```python
from build123d import *

# Parameters (mm, degrees)
F1_DEPTH  = 127
F2_R      = 16.6289302691
F3_DEPTH  = 6.35
F4_W      = 2.8006685898
F4_H      = 13.494130224
F4_W_2    = 2.8006681241
F4_H_2    = 14.0033438802
F5_DEPTH  = 2.54
F6_R      = 6.3651576638
F7_DEPTH  = 3.81
F10_W     = 45.3136
F10_H     = 30.0435274839
F11_DEPTH = 1.27


# Not quite as in the source:
# - a feature of the source that left no trace in its solid (it failed there, or was rolled back) is left out


with BuildPart() as f1:
    # F0 (on Top) → F1 (new body)
    with BuildSketch(Plane.XY):
        with BuildLine():
            ThreePointArc((24.3542956412, 0), (-7.3957043588, 15.8499764569), (-39.1457043588, 0))
            Line((-39.1457043588, 0), (24.3542956412, 0))
        make_face()
    extrude(amount=F1_DEPTH)

    # F2 (on face) → F3 (join)
    with BuildSketch(Plane.XZ):
        with Locations((-6.1257043588, 43.7316484749)):
            Circle(F2_R)
    extrude(amount=F3_DEPTH)

    # F4 (on face) → F5 (join)
    with BuildSketch(Plane.XZ.offset(6.35)):
        with Locations((-15.4036753811, 41.3128901273)):
            Rectangle(F4_W, F4_H)
        with Locations((1.4003340621, 41.0582832992)):
            Rectangle(F4_W_2, F4_H_2)
    extrude(amount=-F5_DEPTH)

    # F6 (on face) → F7 (join)
    with BuildSketch(Plane.XZ.offset(6.35)):
        with Locations((-7.1289734915, 40.9309826791)):
            Circle(F6_R)
    extrude(amount=F7_DEPTH)

    # F10 (on face) → F11 (join)
    with BuildSketch(Plane.XZ):
        with Locations((-8.6597625557, 100.2542302012)):
            Rectangle(F10_W, F10_H)
    extrude(amount=F11_DEPTH)


solid = f1.part
```
Work out the finished part from the listing and answer in its coordinate system (mm). A direction names the side the tool comes from. Round coordinates to 2 decimals unless told otherwise and drop trailing zeros. Write each loop counter-clockwise with the first axis right and the second up, starting at its lowest first coordinate (ties: lowest second). Pieces come first, ordered by that corner, then holes. Notation, with made-up numbers: (66, -29.5) - (85, -29.5) arc R37 cw to (85, 7.5) - close; hole circle Ø6 at (8.25, 61). An arc over 180 degrees is marked (long way). Return JSON: item names as keys, results as strings. Group by question number.
Q1. Find the intervals of material crossed by L1, parallel to X at y = -5, z = 43.5; L2, parallel to Z at x = -9.5, y = -4.5; L3, parallel to X at y = 11.25, z = 104, in increasing order.
Q2. For faces 5 (the flat face through (-9, -1.27, 100)), 6 (the cylindrical face through (-9.73, -3.13, 27.5)), 7 (the cylindrical face through (-6.881, 15.847, 62.611)), determine the directions among +Z, -Z, +X, -X, +Y, -Y from which every point of the face is accessible in a straight line to the end or side of a thin tool.
Q3. The part is cut by section C-C on y = 7. Write down the section's boundary in (x, z).
Q4. Each of these flat-tipped pins is pushed along its axis until it touches: pin 1 Ø2 at (x, z) = (15, 45) entering from -Y; pin 2 Ø1.5 at (y, z) = (5.5, 93) entering from +X; pin 3 Ø1 at (x, y) = (9, -6.5) entering from -Z. Where does it stop, or does it pass through?
Q5. The part is cut by section B-B on x = -11. Write down the section's boundary in (y, z).
Q6. The part is cut by section D-D on x = -27. Write down the section's boundary in (y, z), then the cut area to 3 significant figures.
Q7. The part is cut by section A-A on z = 106. Write down the section's boundary in (x, y).
Q8. The mould has two halves that part along Z. Classify faces 1 (the flat face through (-8, 6, 127)), 2 (the flat face through (-6, -6.35, 48)), 3 (the flat face through (-8, 0, 63)), 4 (the cylindrical face through (-7.96, -8.23, 47.24)): released by +Z, released by -Z, zero draft, split by the parting line, or undercut.
Solved:
{
 "1": {"L1": "-22.75 to 10.5", "L2": "27.45 to 60.01", "L3": "-25.95 to 11.16"},
 "2": {"face 5": "+Z, +X, -X, -Y", "face 6": "-Y", "face 7": "+Z, -Z, +Y"},
 "3": {"outline": "(-32.39, 0) - (17.6, 0) - (17.6, 127) - (-32.39, 127) - close"},
 "4": {"pin 1": "y = 0", "pin 2": "x = 20.15", "pin 3": "z = 35.86"},
 "5": {"outline": "(-10.16, 35.88) - (-6.35, 35.88) - (-6.35, 27.83) - (0, 27.83) - (0, 0) - (15.69, 0) - (15.69, 127) - (0, 127) - (0, 115.28) - (-1.27, 115.28) - (-1.27, 85.23) - (0, 85.23) - (0, 59.63) - (-6.35, 59.63) - (-6.35, 45.98) - (-10.16, 45.98) - close"},
 "6": {"outline": "(-1.27, 85.23) - (0, 85.23) - (0, 0) - (10.68, 0) - (10.68, 127) - (0, 127) - (0, 115.28) - (-1.27, 115.28) - close", "area": "1,390 mm²"},
 "7": {"outline": "(-39.15, 0) - (-31.32, 0) - (-31.32, -1.27) - (14, -1.27) - (14, 0) - (24.35, 0) arc R39.73 ccw to start"},
 "8": {"face 1": "released by +Z", "face 2": "zero draft", "face 3": "undercut", "face 4": "split by the parting line"}
}
